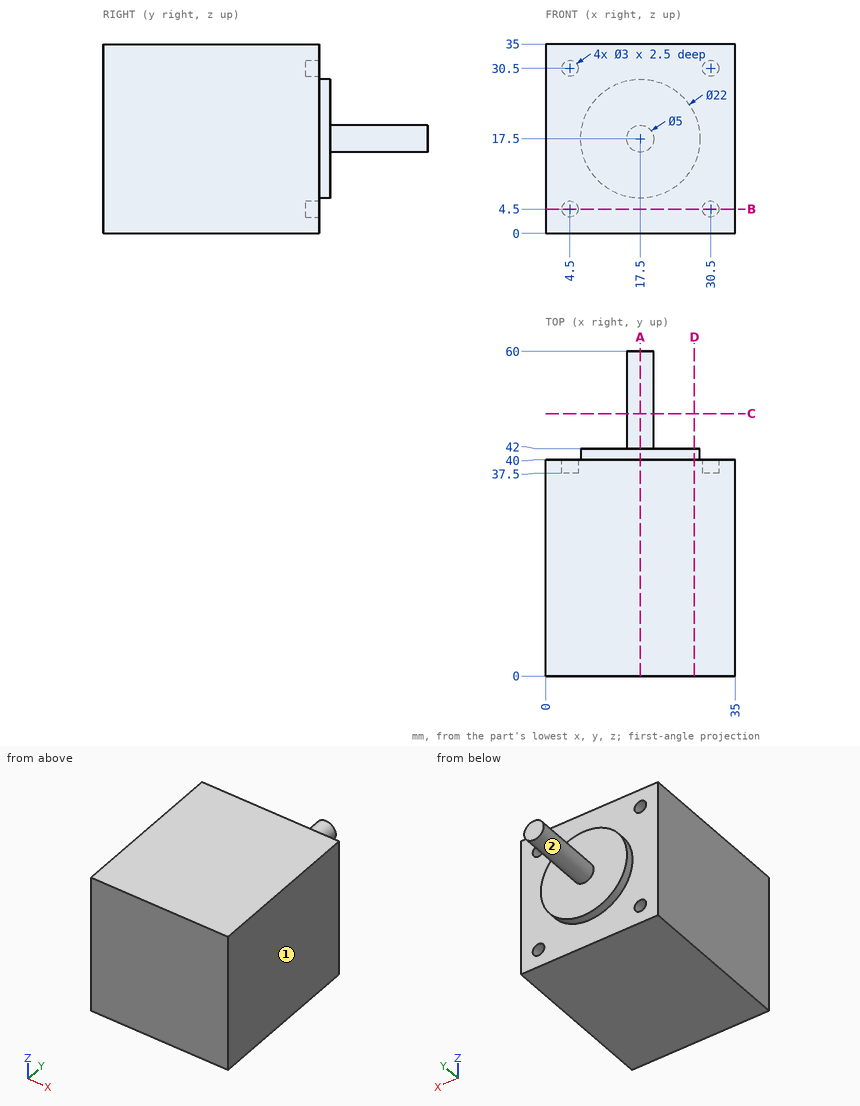
Can you work these out from the drawing? Everything is in mm from the part's minimum corner. A direction names the side the tool comes from. Coordinates: 2 decimals unless noted, no trailing zeros. Loops run counter-clockwise (first coordinate to the right, second up) from the corner with the lowest first, then second, coordinate; pieces in that order, holes last. Notation, with made-up numbers: M 73.5,-5.5 L 126.5,-5.5 A7 cw 126.5,0.5 Z; hole C -32.5,14 d2. An arc over 180 degrees is marked long. Put each result on its own line as item: value. Start each with the question number.
(1) Suppose I cut it at A-A on x = 17.5. Please give me the cut outline in (y, z).
(2) Suppose I cut it at D-D on x = 27.5. Please give me the cut outline in (y, z).
(3) Suppose I cut it at B-B on z = 4.5. Please give me the cut outline in (x, y).
(4) For the marked faces 1 and 2, which set-ups out of +Z, -Z, +X, -X, +Y, -Y let a thin tool reach every point of the face, with its end or its side?
(5) Suppose I cut it at C-C on y = 48.5. Please give me the cut outline in (x, z).
(6) I need wall thicknesses on line 1 (X direction, y = 38.3, z = 30.5); line 2 (X direction, y = 39, z = 4). Which ranges of each line are inside material? Lowest first, please. Write a range as from..to.
(7) Will these pins go through, and if not, where does the flat tip stop? P1, Ø1.5, axis at x = 4.5, z = 30.5, coming from the +Y side; P2, Ø1, axis at x = 5.5, z = 21.5, coming from the +Y side; P3, Ø12, axis at x = 26.5, y = 47, coming from the -Z side; P4, Ø3, axis at y = 44, z = 12.5, coming from the +X side.
Solutions:
1. outline: M 0,0 L 40,0 L 40,6.5 L 42,6.5 L 42,15 L 60,15 L 60,20 L 42,20 L 42,28.5 L 40,28.5 L 40,35 L 0,35 Z
2. outline: M 0,0 L 40,0 L 40,12.92 L 42,12.92 L 42,22.08 L 40,22.08 L 40,35 L 0,35 Z
3. outline: M 0,0 L 35,0 L 35,40 L 32,40 L 32,37.5 L 29,37.5 L 29,40 L 6,40 L 6,37.5 L 3,37.5 L 3,40 L 0,40 Z
4. face 1: +Z, -Z, +X, +Y, -Y
4. face 2: +Y
5. outline: C 17.5,17.5 d5
6. line 1: x = 0..3, 6..29, 32..35
6. line 2: x = 0..3.09, 5.91..29.09, 31.91..35
7. P1: stops at y = 37.5
7. P2: stops at y = 40
7. P3: stops at z = 8.08
7. P4: passes through
